Build history of the part. All positions in model axes, mm. Coordinates: 2 decimals unless noted, no trailing zeros. Write each loop counter-clockwise with the first axis right and the second up, starting at its lowest first coordinate (ties: lowest second). Pieces come first, ordered by that corner, then holes.
Autodesk Inventor part; units mm, degrees
ref_plane "YZ Plane" through (0, 0, 0) normal (1, 0, 0) x (0, 1, 0)
ref_plane "XZ Plane" through (0, 0, 0) normal (0, 1, 0) x (-1, 0, 0)
ref_plane "XY Plane" through (0, 0, 0) normal (0, 0, 1) x (1, 0, 0)
sketch "Sketch1" plane through (0, 0, 0) normal (0, 0, 1) x (1, 0, 0)
  line L0 (105.0559, -3.8299) -> (47.0396, -3.8299)
  line L1 (47.0396, -3.8299) -> (47.0396, -56.241)
  line L2 (47.0396, -56.241) -> (105.0559, -56.241)
  line L3 (105.0559, -56.241) -> (105.0559, -3.8299)
  point P0 (0, 0)
extrude "Extrusion1" add sketch "Sketch1" along normal blind 46.0375 and the other way blind 23.8252
chamfer "Chamfer1" distance 31.75 angle 45 1 edges at (47.0396, -30.0355, -23.8252)
chamfer "Chamfer2" distance 31.75 angle 45 1 edges at (105.0559, -30.0355, 46.0375)
sketch "Sketch2" plane through (0, 0, 46.0375) normal (0, 0, 1) x (1, 0, 0)
  circle A0 centre (63.8131, -28.5354) radius 10
  point P0 (0, 0)
  dimension "d11" = 20
extrude "Extrusion2" cut sketch "Sketch2" against normal through all
properties part number "MotorCarrier"
1. Flat gauge pins, fed straight in: pin 1 (6 mm diameter, centred on x = 78.5, y = -46.5, fed in from +Z); pin 2 (3 mm diameter, centred on y = -46.5, z = 36.5, fed in from +X). Where does each tip first touch, or does it go through?
Computed values:
pin 1: stops at z = 43.84
pin 2: stops at x = 84.34
2. Saw through at C-C on z = 2.5. List the corners of the cut face in (x, y), plus the area to 3 significant figures.
Computed values:
outline: (52.46, -56.24) - (105.06, -56.24) - (105.06, -3.83) - (52.46, -3.83) - close; hole circle Ø20 at (63.81, -28.54)
area: 2,440 mm2
3. Saw through at B-B on y = -51. List the corners of the cut face in (x, z).
Computed values:
outline: (47.04, 7.92) - (78.79, -23.83) - (105.06, -23.83) - (105.06, 14.29) - (73.31, 46.04) - (47.04, 46.04) - close
4. Saw through at A-A on y = -21. List the corners of the cut face in (x, z).
Computed values:
outline: (47.04, 7.92) - (57.24, -2.27) - (57.24, 46.04) - (47.04, 46.04) - close; (70.39, -15.42) - (78.79, -23.83) - (105.06, -23.83) - (105.06, 14.29) - (73.31, 46.04) - (70.39, 46.04) - close
5. Saw through at D-D on z = -6. List the corners of the cut face in (x, y).
Computed values:
outline: (60.96, -56.24) - (105.06, -56.24) - (105.06, -3.83) - (60.96, -3.83) - (60.96, -18.95) arc R10 cw (long way) to (60.96, -38.12) - close
6. Mould opens along X. For faces 1 (the face through (73.35, -25.53, 21.26)), 2 (the face through (76, -56.241, 11)), 3 (the face through (89.403, -30.402, 29.94)) say: +X half, -X half, draft (parallel to the pull), parting line (faces both ways), or undercut.
Computed values:
face 1: undercut
face 2: draft
face 3: +X half
7. Probe line 1 along Y through (x, z) = (72, 39.5); line 2 along Y through (x, z) = (70, 17); line 3 along X through (y, z) = (-20, 37.5). List the from-to ranges inside material, lowest first.
Computed values:
line 1: y = -56.24 to -34.28, -22.79 to -3.83
line 2: y = -56.24 to -36.39, -20.68 to -3.83
line 3: x = 47.04 to 58.6, 69.02 to 81.84
